Could you check a few things on this drawing? It's one solid part, dimensions in mm from its lowest x, y, z. A direction names the side the tool comes from. Coordinates: 2 decimals unless noted, no trailing zeros. Order: outer loops, then holes, each group sorted by start corner. A loop starts at its lowest first (then second) coordinate and runs counter-clockwise, first axis right, second up.
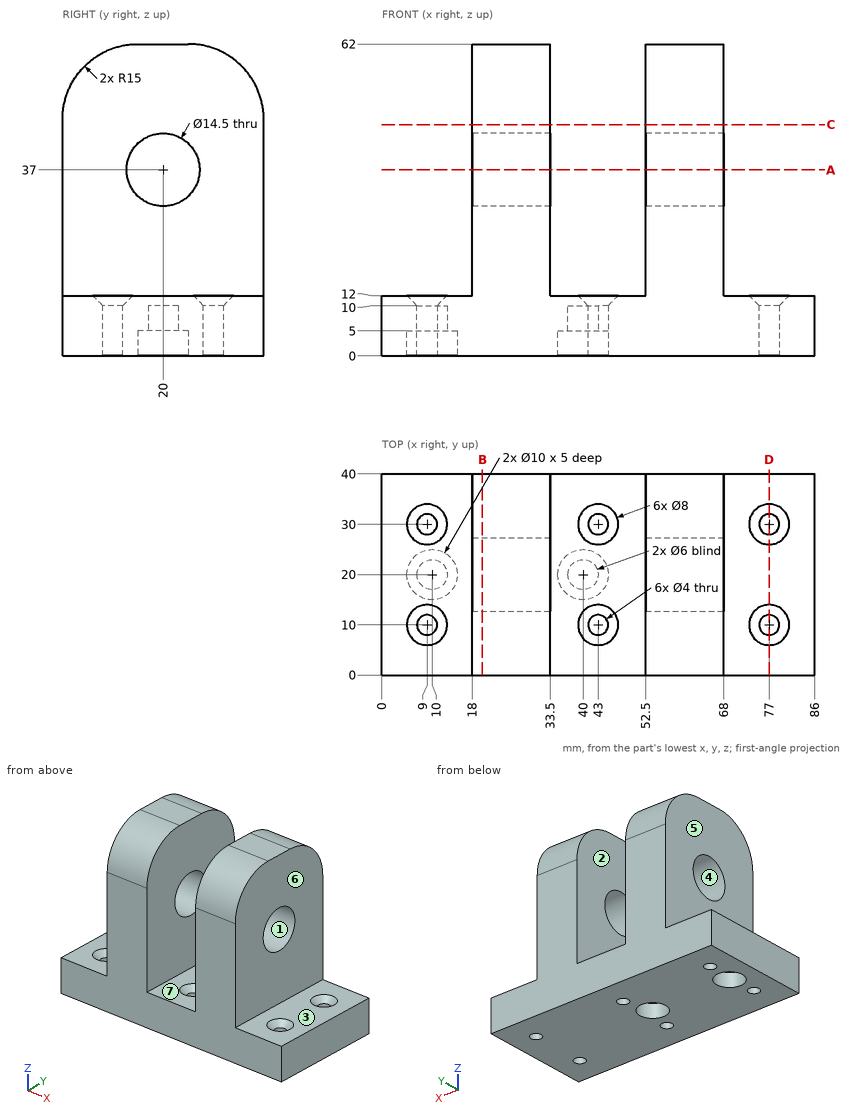
Q1. If we section it at A-A on z = 37: Write out the boundary of the cut face in (x, y).
Q2. If we section it at C-C on z = 46: Write out the boundary of the cut face in (x, y).
Q3. If we section it at B-B on x = 20: Write out the boundary of the cut face in (y, z).
Q4. For the marked faces 5, 6 and 7, which set-ups out of +Z, -Z, +X, -X, +Y, -Y let a thin tool reach every point of the face, with its end or its side?
Q5. We'd pull the mould along Z, two halves only. Please class the marked faces 1, 2, 3 and 4: pulls with the +Z half, pulls with the -Z half, needs draft (parallel to the pull), parting line crosses it, or undercut.
Q6. If we section it at D-D on x = 77: Write out the boundary of the cut face in (y, z), then the cut area to 3 significant figures.
Q7. Will these pins go through, and if not, where does the flat tip stop? pin 1 (10 mm diameter, centred on y = 17.5, z = 20.5, fed in from +X); pin 2 (10 mm diameter, centred on x = 10.5, z = 36.5, fed in from -Y); pin 3 (5 mm diameter, centred on x = 9, y = 30, fed in from +Z); pin 4 (12 mm diameter, centred on y = 29.5, z = 53.5, fed in from -X).
Q8. I need wall thicknesses on L1, parallel to Y at x = 77, z = 8.25; L2, parallel to X at y = 37, z = 55; L3, parallel to Z at x = 39, y = 25.5. Which ranges of each line are inside material? Lowest first, please.
Reply:
1. outline: (18, 0) - (33.5, 0) - (33.5, 12.75) - (18, 12.75) - close; (18, 27.25) - (33.5, 27.25) - (33.5, 40) - (18, 40) - close; (52.5, 0) - (68, 0) - (68, 12.75) - (52.5, 12.75) - close; (52.5, 27.25) - (68, 27.25) - (68, 40) - (52.5, 40) - close
2. outline: (18, 0) - (33.5, 0) - (33.5, 40) - (18, 40) - close; (52.5, 0) - (68, 0) - (68, 40) - (52.5, 40) - close
3. outline: (0, 0) - (40, 0) - (40, 47) arc R15 ccw to (25, 62) - (15, 62) arc R15 ccw to (0, 47) - close; hole circle Ø14.5 at (20, 37)
4. face 5: +Z, -X, +Y, -Y
4. face 6: +Z, +X, +Y, -Y
4. face 7: +Z, +Y, -Y
5. face 1: undercut
5. face 2: needs draft
5. face 3: pulls with the +Z half
5. face 4: undercut
6. outline: (0, 0) - (8, 0) - (8, 10) - (6, 12) - (0, 12) - close; (12, 0) - (28, 0) - (28, 10) - (26, 12) - (14, 12) - (12, 10) - close; (32, 0) - (40, 0) - (40, 12) - (34, 12) - (32, 10) - close
6. area: 376 mm2
7. pin 1: stops at x = 68
7. pin 2: passes through
7. pin 3: stops at z = 10.5
7. pin 4: stops at x = 18
8. L1: y = 0 to 8, 12 to 28, 32 to 40
8. L2: x = 18 to 33.5, 52.5 to 68
8. L3: z = 0 to 12
